Design review of the part shown in the three views and the two pictorial views. Dimensions are in mm from the part's minimum x, y and z. A direction names the side the tool comes from. Give positions to 0.01 mm unless a question says otherwise; leave off trailing zeros. Loops run counter-clockwise (first coordinate to the right, second up) from the corner with the lowest first, then second, coordinate; pieces in that order, holes last.
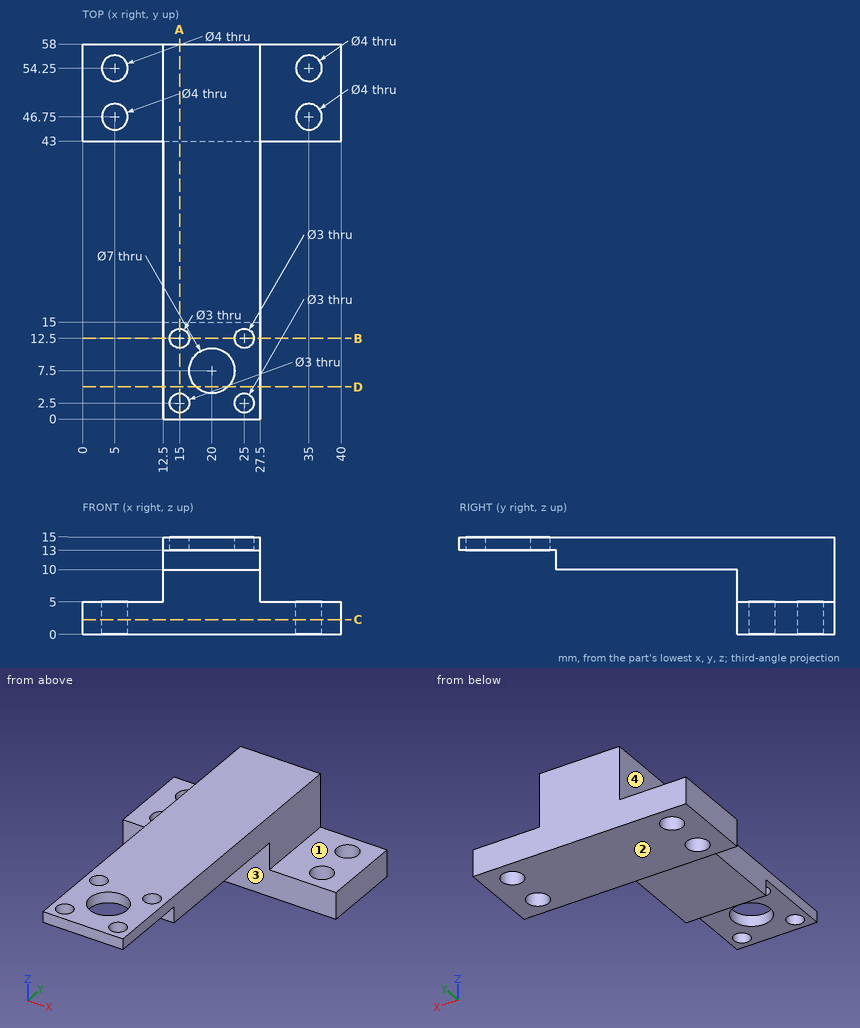
Q1. Take a section at B-B (y = 12.5). Give the boundary of the cut face in (x, z).
Results:
outline: (12.5, 13) - (13.5, 13) - (13.5, 15) - (12.5, 15) - close; (16.5, 13) - (23.5, 13) - (23.5, 15) - (16.5, 15) - close; (26.5, 13) - (27.5, 13) - (27.5, 15) - (26.5, 15) - close
Q2. Wall thickness on line 1 (Y direction, x = 20, z = 14.6); line 2 (Y direction, x = 5, z = 1.7); line 3 (Z direction, x = 10, y = 51): over which ranges is each line inside the solid? List them lowest first.
Results:
line 1: y = 0 to 4, 11 to 58
line 2: y = 43 to 44.75, 48.75 to 52.25, 56.25 to 58
line 3: z = 0 to 5
Q3. Take a section at A-A (x = 15). Give the boundary of the cut face in (y, z).
Results:
outline: (0, 13) - (1, 13) - (1, 15) - (0, 15) - close; (4, 13) - (11, 13) - (11, 15) - (4, 15) - close; (14, 13) - (15, 13) - (15, 10) - (43, 10) - (43, 0) - (58, 0) - (58, 15) - (14, 15) - close
Q4. Take a section at D-D (y = 5). Give the boundary of the cut face in (x, z).
Results:
outline: (12.5, 13) - (17.55, 13) - (17.55, 15) - (12.5, 15) - close; (22.45, 13) - (27.5, 13) - (27.5, 15) - (22.45, 15) - close
Q5. Take a section at C-C (z = 2.25). Give the boundary of the cut face in (x, y).
Results:
outline: (0, 43) - (40, 43) - (40, 58) - (0, 58) - close; hole circle Ø4 at (5, 46.75); hole circle Ø4 at (5, 54.25); hole circle Ø4 at (35, 46.75); hole circle Ø4 at (35, 54.25)
Q6. Tool access review of the marked faces 1, 2, 3 and 4: name each direction out of +Z, -Z, +X, -X, +Y, -Y from which nothing blocks a thin tool from reaching the whole face with its end or side.
Results:
face 1: +Z, +X, +Y, -Y
face 2: -Z, +X, -X, +Y, -Y
face 3: -Z, +X, -X, -Y
face 4: +Z, -X, +Y, -Y
Q7. Insertion check: pin 1 (6.5 mm diameter, centred on x = 20, y = 7.5, fed in from -Z); pin 2 (16.5 mm diameter, centred on x = 23, y = 26, fed in from -Z); pin 3 (10 mm diameter, centred on x = 6.5, y = 47, fed in from +Z); pin 4 (1.5 mm diameter, centred on x = 18.5, z = 10, fed in from -Y). Each pin has a flat end and moves straight along its axis. Give the tip position at first contact, or say it passes through.
Results:
pin 1: passes through
pin 2: stops at z = 10
pin 3: stops at z = 5
pin 4: stops at y = 15
